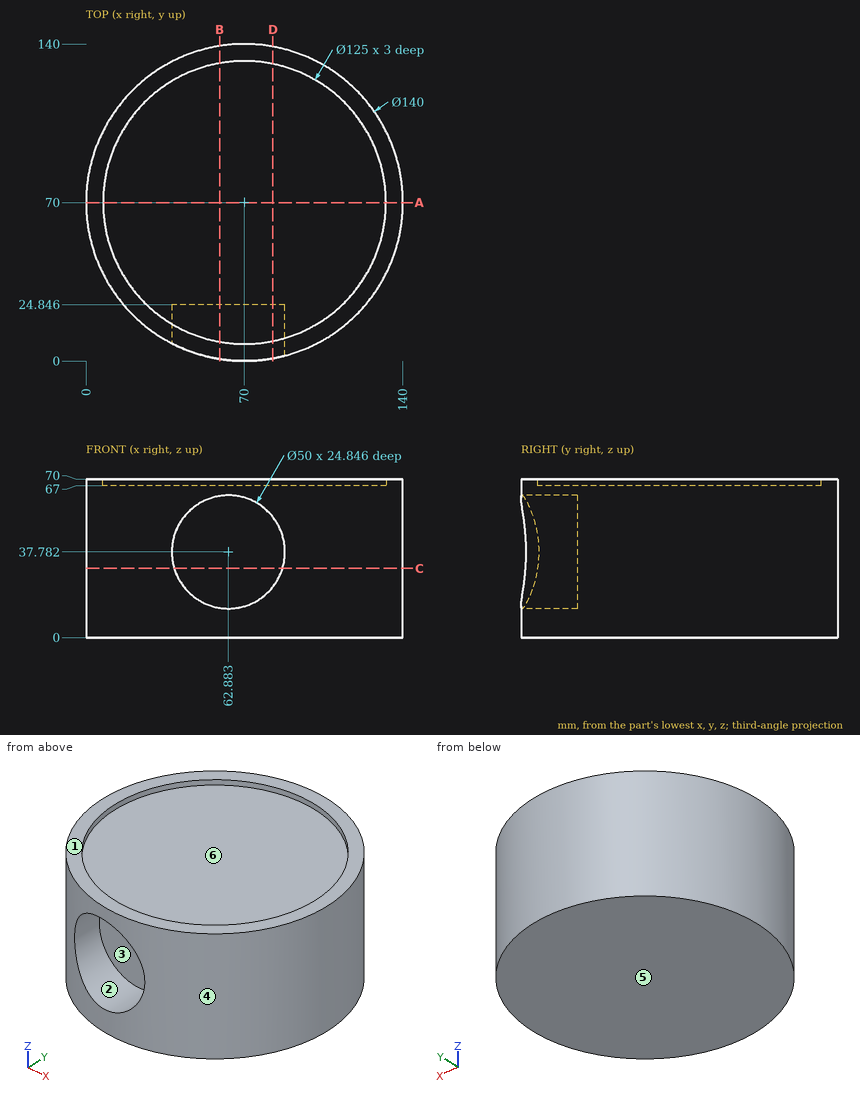
Study the drawing (mm; zero at the part's minimum x, y, z) and answer. A direction names the side the tool comes from. Give positions to 0.01 mm unless a question says otherwise; leave off trailing zeros. Write each loop counter-clockwise with the first axis right and the second up, starting at its lowest first coordinate (ties: lowest second). Pieces come first, ordered by that corner, then holes.
Item 1: Find the intervals of material crossed by line 1 along Y through (x, z) = (70, 68); line 2 along Z through (x, y) = (71.5, 131); line 3 along X through (y, z) = (68, 22), in increasing order.
Item 2: Determine the mould class of the marked faces 1, 2, 3 and 4 for opening direction X: released by +X, released by -X, zero draft, split by the parting line, or undercut.
Item 3: Section A-A, the plane y = 70 is taken. Write down the section's boundary in (x, z), plus the area to 4 significant figures.
Item 4: Flat-ended cylindrical pins translate along their axes: P1, Ø1, axis at x = 47.5, y = 101, coming from the +Z side; P2, Ø5, axis at y = 27.5, z = 29, coming from the +X side (1 decimal); P3, Ø15, axis at x = 51.5, z = 30.5, coming from the -Y side. Find the tip coordinate at first contact, or state that the pin passes through.
Item 5: Which of the six approach directions +Z, -Z, +X, -X, +Y, -Y give full straight-line access (tool end or side, diameter ignored) to the marked faces 5 and 6?
Item 6: Section C-C, the plane z = 30.5 is taken. Write down the section's boundary in (x, y) (1 decimal).
Item 7: Section D-D, the plane x = 82.5 is taken. Write down the section's boundary in (y, z) (1 decimal), plus the area to 3 significant figures.
Item 8: Section B-B, the plane x = 59 is taken. Write down the section's boundary in (y, z) (1 decimal).
Completed:
1. line 1: y = 0 to 7.5, 132.5 to 140
1. line 2: z = 0 to 67
1. line 3: x = 0.03 to 139.97
2. face 1: zero draft
2. face 2: undercut
2. face 3: undercut
2. face 4: split by the parting line
3. outline: (0, 0) - (140, 0) - (140, 70) - (132.5, 70) - (132.5, 67) - (7.5, 67) - (7.5, 70) - (0, 70) - close
3. area: 9,425 mm2
4. P1: stops at z = 67
4. P2: stops at x = 127.4
4. P3: stops at y = 24.85
5. face 5: -Z, +X, -X, +Y, -Y
5. face 6: +Z
6. outline: (39, 7.3) - (39, 24.8) - (86.8, 24.8) - (86.8, 2) arc R70 ccw (long way) to start
7. outline: (1.1, 0) - (138.9, 0) - (138.9, 70) - (131.2, 70) - (131.2, 67) - (8.8, 67) - (8.8, 70) - (1.1, 70) - (1.1, 53.3) - (24.8, 53.3) - (24.8, 22.3) - (1.1, 22.3) - close
7. area: 8,540 mm2
8. outline: (0.9, 0) - (139.1, 0) - (139.1, 70) - (131.5, 70) - (131.5, 67) - (8.5, 67) - (8.5, 70) - (0.9, 70) - (0.9, 62.5) - (24.8, 62.5) - (24.8, 13.1) - (0.9, 13.1) - close
